Read the model definition and answer for the solid it produces. Units are mm, in the model's axes. A direction names the side the tool comes from. Give positions to 0.01 mm unless a question says otherwise; leave off trailing zeros. Order: outer loops, then holes, each group sorted by start corner. A loop starts at its lowest first (then second) coordinate and runs counter-clockwise, first axis right, second up.
```python
from build123d import *

# Parameters (mm, degrees)
BOSS_EXTRU_1_DEPTH = 70
SKETCH1_R          = 2
CUT_EXTRUDE1_DEPTH = 10


with BuildPart() as part:
    # Esquisse1 → Boss.-Extru.1 (new body)
    with BuildSketch(Plane.XY):
        with BuildLine():
            Line((-10.5, 0), (10.5, 0))
            Line((10.5, 0), (11.996134815, 2.600303947))
            ThreePointArc((11.996134815, 2.600303947), (13.310550199, 3.611999394), (13.524605519, 5.256808137))
            Line((13.524605519, 5.256808137), (14.524605519, 5.256808137))
            ThreePointArc((14.524605519, 5.256808137), (14.624387393, 3.298979885), (13.310550199, 1.844029812))
            Line((13.310550199, 1.844029812), (11.249883314, -1))
            Line((11.249883314, -1), (-11.750116686, -1))
            Line((-11.750116686, -1), (-13.310550199, 1.844029812))
            ThreePointArc((-13.310550199, 1.844029812), (-14.624387393, 3.298979885), (-14.524605519, 5.256808137))
            Line((-14.524605519, 5.256808137), (-13.524605519, 5.256808137))
            ThreePointArc((-13.524605519, 5.256808137), (-13.310550199, 3.611999394), (-11.996134815, 2.600303947))
            Line((-11.996134815, 2.600303947), (-10.5, 0))
        make_face()
    extrude(amount=BOSS_EXTRU_1_DEPTH)

    # Sketch1 → Cut-Extrude1 (cut)
    with BuildSketch(Plane.XZ.offset(1)):
        with Locations(Location((-1.130377356, 49.868372079, 0), (0, 0, 270))):
            Circle(SKETCH1_R)
    extrude(amount=-CUT_EXTRUDE1_DEPTH, mode=Mode.SUBTRACT)


solid = part.part
```
1) A tool of negligible diameter and unlimited length cuts with its end or side. For faces 1 (the face through (-13.32, 3.63, 34.51)), 2 (the face through (-11.26, 1.32, 34.51)), 3 (the face through (12.295, 0.442, 34.51)), from which of +Z, -Z, +X, -X, +Y, -Y can it reach the whole face along a straight path? Write none if from no direction.
Final values:
face 1: +Z, -Z
face 2: +Z, -Z, +Y
face 3: +Z, -Z, +X, -Y
2) The part is cut by section D-D on x = 9. Determine the outline of the cut face in (y, z), and give its area (3 significant figures).
Final values:
outline: (-1, 0) - (0, 0) - (0, 70) - (-1, 70) - close
area: 70.0 mm2
3) The part is cut by section C-C on z = 7.5. Determine the outline of the cut face in (x, y).
Final values:
outline: (-14.52, 5.26) arc R2.56 ccw to (-13.31, 1.84) - (-11.75, -1) - (11.25, -1) - (13.31, 1.84) arc R2.56 ccw to (14.52, 5.26) - (13.52, 5.26) arc R2.17 cw to (12, 2.6) - (10.5, 0) - (-10.5, 0) - (-12, 2.6) arc R2.17 cw to (-13.52, 5.26) - close
4) For a pull along X with two mould halves and no side action, classify faces 4 (the face through (0, 0, 35)), 5 (the face through (-12.52, 0.4, 34.51)), 6 (the face through (0.1, -0.2, 70)) as released by +X, released by -X, zero draft, split by the parting line, or undercut.
Final values:
face 4: undercut
face 5: released by -X
face 6: zero draft
5) The part is cut by section A-A on x = -0.5. Determine the outline of the cut face in (y, z).
Final values:
outline: (-1, 0) - (0, 0) - (0, 47.97) - (-1, 47.97) - close; (-1, 51.77) - (0, 51.77) - (0, 70) - (-1, 70) - close
6) Consider L1, parallel to Y at x = -5.5, z = 60; L2, parallel to X at y = 2.5, z = 32; L3, parallel to X at y = 0.5, z = 29. Determine where each line is inside the solid, lowest interval first.
Final values:
L1: y = -1 to 0
L2: x = -14.16 to -11.94, 11.94 to 14.16
L3: x = -12.57 to -10.79, 10.79 to 12.34
7) The part is cut by section B-B on y = 4.5. Determine the outline of the cut face in (x, z).
Final values:
outline: (-14.75, 0) - (-13.59, 0) - (-13.59, 70) - (-14.75, 70) - close; (13.59, 0) - (14.75, 0) - (14.75, 70) - (13.59, 70) - close
8) Given pin 1 (6.5 mm diameter, centred on x = 0.5, z = 37.5, fed in from +Y), flat-ended and moving along its own axis, determine where the tip first touches the part or whether it passes through.
Final values:
pin 1: stops at y = 0
